Work out the finished part from the listing and answer in its coordinate system (mm). A direction names the side the tool comes from. Give positions to 0.01 mm unless a question says otherwise; leave off trailing zeros. Loops run counter-clockwise (first coordinate to the right, second up) from the corner with the lowest first, then second, coordinate; pieces in that order, holes last.
from build123d import *

# Parameters (mm, degrees)
SKETCH_1_R          = 100
EXTRUDE_1_DEPTH     = 30
SKETCH_2_R          = 75
EXTRUDE_2_DEPTH     = 120
SKETCH_3_R          = 40
CUT_EXTRUDE_1_DEPTH = 186.47236991
SKETCH_4_R          = 8
CUT_EXTRUDE_2_DEPTH = 186.47236991
CHAMFER_1_SIZE      = 5


with BuildPart() as part:
    # 草图1 → 凸台-拉伸1 (new body)
    with BuildSketch(Plane.XY):
        Circle(SKETCH_1_R)
    extrude(amount=EXTRUDE_1_DEPTH)

    # 草图2 → 凸台-拉伸2 (add)
    with BuildSketch(Plane.XY):
        Circle(SKETCH_2_R)
    extrude(amount=EXTRUDE_2_DEPTH)

    # 草图3 → 切除-拉伸1 (cut, through all)
    with BuildSketch(Plane.XY):
        Circle(SKETCH_3_R)
    extrude(amount=CUT_EXTRUDE_1_DEPTH, mode=Mode.SUBTRACT)

    # 草图4 → 切除-拉伸2 (cut, through all)
    with BuildSketch(Plane.XY):
        with Locations((87, 0)):
            Circle(SKETCH_4_R)
        with Locations((61.518289963, 61.518289963)):
            Circle(SKETCH_4_R)
        with Locations((0, 87)):
            Circle(SKETCH_4_R)
        with Locations((-61.518289963, 61.518289963)):
            Circle(SKETCH_4_R)
        with Locations((-87, 0)):
            Circle(SKETCH_4_R)
        with Locations((-61.518289963, -61.518289963)):
            Circle(SKETCH_4_R)
        with Locations((0, -87)):
            Circle(SKETCH_4_R)
        with Locations((61.518289963, -61.518289963)):
            Circle(SKETCH_4_R)
    extrude(amount=CUT_EXTRUDE_2_DEPTH, mode=Mode.SUBTRACT)

    # 倒角1
    chamfer_1_edges = [part.edges().sort_by_distance(p)[0] for p in [
        (-40, 0, 120),
    ]]
    chamfer(chamfer_1_edges, length=CHAMFER_1_SIZE)


solid = part.part
Item 1: Find section D-D, the plane y = 87. Write down the section's boundary in (x, z).
Item 2: Find section A-A, the plane x = 0. Write down the section's boundary in (y, z).
Item 3: Consider line 1 (X direction, y = -56, z = 24.5); line 2 (X direction, y = 0, z = 37); line 3 (Z direction, x = 81, y = -40.5). Determine where each line is inside the solid, lowest interval first.
Item 4: For faces 4 (the face through (-9.764, 74.362, 74.37)), 5 (the face through (32, -32, 120)), determine the directions among +Z, -Z, +X, -X, +Y, -Y from which every point of the face is accessible in a straight line to the end or side of a thin tool.
Item 5: Flat-ended cylindrical pins translate along their axes: pin 1 Ø2 at (x, z) = (51.5, 22.5) entering from -Y; pin 2 Ø21 at (x, y) = (0, -87) entering from +Z; pin 3 Ø2 at (x, z) = (52, 63.5) entering from +Y. Find the tip coordinate at first contact, or state that the pin passes through.
Item 6: Find section C-C, the plane x = 86.5. Write down the section's boundary in (y, z), plus the area to 3 significant figures.
Item 7: Determine the mould class of faces 1 (the face through (95.38, 30.04, 14.79)), 2 (the face through (-15, -74, 30)), 3 (the face through (55.622, -56.112, 14.79)) for opening direction X: released by +X, released by -X, zero draft, split by the parting line, or undercut.
Ans:
1. outline: (-49.31, 0) - (-8, 0) - (-8, 30) - (-49.31, 30) - close; (8, 0) - (49.31, 0) - (49.31, 30) - (8, 30) - close
2. outline: (-100, 0) - (-95, 0) - (-95, 30) - (-100, 30) - close; (-79, 0) - (-40, 0) - (-40, 115) - (-45, 120) - (-75, 120) - (-75, 30) - (-79, 30) - close; (40, 0) - (79, 0) - (79, 30) - (75, 30) - (75, 120) - (45, 120) - (40, 115) - close; (95, 0) - (100, 0) - (100, 30) - (95, 30) - close
3. line 1: x = -82.85 to -67.31, -55.73 to 55.73, 67.31 to 82.85
3. line 2: x = -75 to -40, 40 to 75
3. line 3: z = 0 to 30
4. face 4: +Z
4. face 5: +Z, +X, -X, +Y, -Y
5. pin 1: stops at y = -86.31
5. pin 2: stops at z = 30
5. pin 3: stops at y = 54.99
6. outline: (-50.18, 0) - (-7.98, 0) - (-7.98, 30) - (-50.18, 30) - close; (7.98, 0) - (50.18, 0) - (50.18, 30) - (7.98, 30) - close
6. area: 2,530 mm2
7. face 1: split by the parting line
7. face 2: zero draft
7. face 3: undercut
